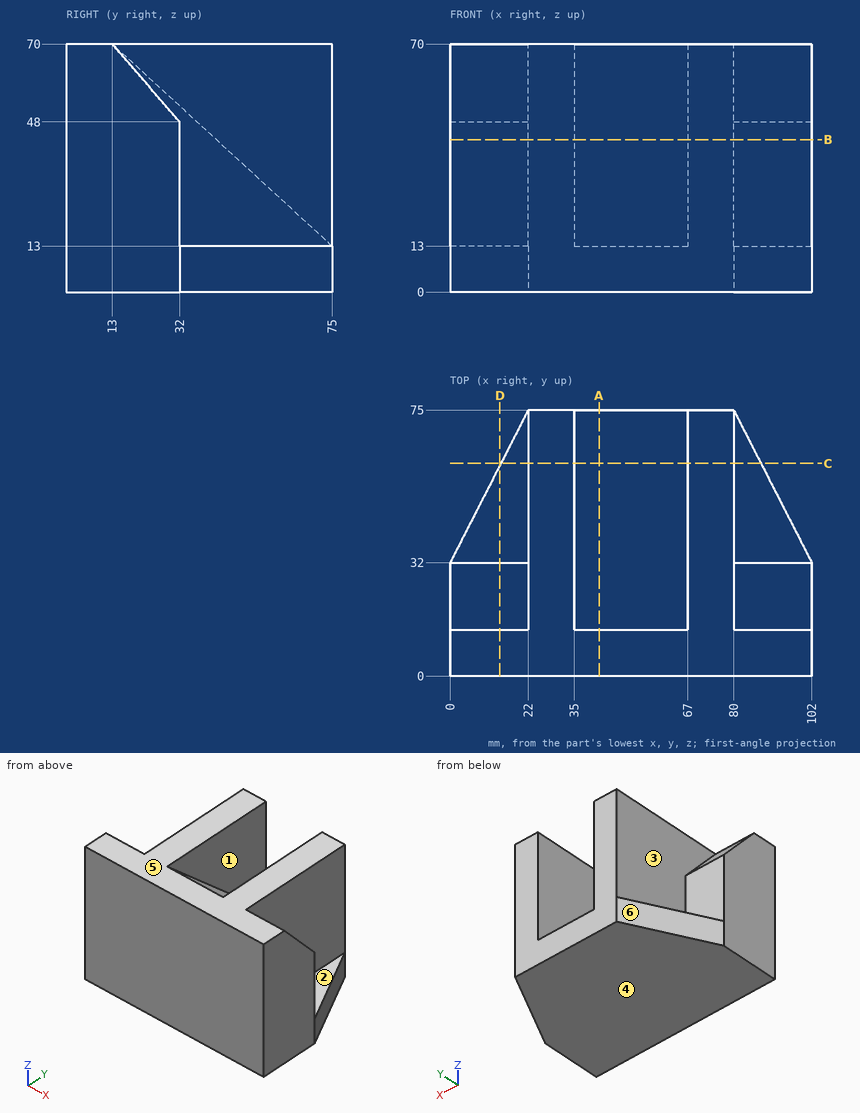
Verification items for this drawing (mm, ordinates from the low corner). A direction names the side the tool comes from. Round coordinates to 2 decimals unless told otherwise and drop trailing zeros. Write each loop counter-clockwise with the first axis right and the second up, starting at its lowest first coordinate (ties: lowest second). Pieces come first, ordered by that corner, then holes. Notation, with made-up numbers: M 33.25,27 L 79.25,27 A9 cw 79.25,31 Z; hole C 46.5,26.5 d7. An arc over 180 degrees is marked long. Write item = value, one per line. Start each with the question number.
1. Release check for a two-part mould opening along Z. For the marked faces 4, 5 and 6 record: pulls with the +Z half, pulls with the -Z half, needs draft (parallel to the pull), parting line crosses it, or undercut.
2. Gauge pin test, flat ends, axial feed: pin 1 (11 mm diameter, centred on x = 87, y = 54.5, fed in from +Z); pin 2 (12 mm diameter, centred on y = 40, z = 10, fed in from +X); pin 3 (6 mm diameter, centred on x = 63, y = 63.5, fed in from +Z); pin 4 (1 mm diameter, centred on x = 68.5, y = 37.5, fed in from -Z). Record the tip position at first contact, or that the pin passes through.
3. Scan lines: line 1 (X direction, y = 53.5, z = 38); line 2 (Y direction, x = 11, z = 27); line 3 (X direction, y = 51, z = 29.5). Record each from-to range of solid material in increasing order. Write a range as [from, to].
4. Section check A-A, the plane x = 42. Record the cut outline in (y, z), then the cut area to 3 significant figures.
5. Section check B-B, the plane z = 43. Record the cut outline in (x, y), then the cut area to 3 significant figures.
6. Tool access check on the marked faces 1, 2 and 3. Record the directions out of +Z, -Z, +X, -X, +Y, -Y that give a thin tool (end or side, any length) a straight path to the whole face; none if there is none.
7. Section check D-D, the plane x = 14. Record the cut outline in (y, z), then the cut area to 3 significant figures.
8. Section check C-C, the plane y = 60. Record the cut outline in (x, z), then the cut area to 3 significant figures.
Results found:
q1.face_4 = pulls with the -Z half
q1.face_5 = pulls with the +Z half
q1.face_6 = needs draft
q2.pin_1 = 13
q2.pin_2 = 100.98
q2.pin_3 = 26.33
q2.pin_4 = 0
q3.line_1 = [22, 35], [67, 80]
q3.line_2 = [0, 32]
q3.line_3 = [22, 80]
q4.outline = M 0,0 L 75,0 L 75,13 L 13,70 L 0,70 Z
q4.area = 3,480 mm^2
q5.outline = M 0,0 L 102,0 L 102,32 L 80,32 L 80,75 L 67,75 L 67,42.37 L 35,42.37 L 35,75 L 22,75 L 22,32 L 0,32 Z
q5.area = 4,710 mm^2
q6.face_1 = +Z, +Y
q6.face_2 = +Z, +X, +Y
q6.face_3 = +Z, -X, +Y
q7.outline = M 0,0 L 59.36,0 L 59.36,13 L 32,13 L 32,48 L 13,70 L 0,70 Z
q7.area = 2,390 mm^2
q8.outline = M 14.33,0 L 87.67,0 L 87.67,13 L 80,13 L 80,70 L 67,70 L 67,26.79 L 35,26.79 L 35,70 L 22,70 L 22,13 L 14.33,13 Z
q8.area = 2,880 mm^2
